Verification items for the finished model (mm, model axes). Face numbers are marked on the shaded views. A direction names the side the tool comes from. Round coordinates to 2 decimals unless told otherwise and drop trailing zeros. Loops run counter-clockwise (first coordinate to the right, second up) from the corner with the lowest first, then second, coordinate; pieces in that order, holes last. Notation, with made-up numbers: (57, -18.75) -> (74, -18.75) arc R4 cw to (74, -14.75) -> close; hole circle Ø4 at (34, -10). An arc over 180 degrees is marked (long way). Write item = value, one per line.
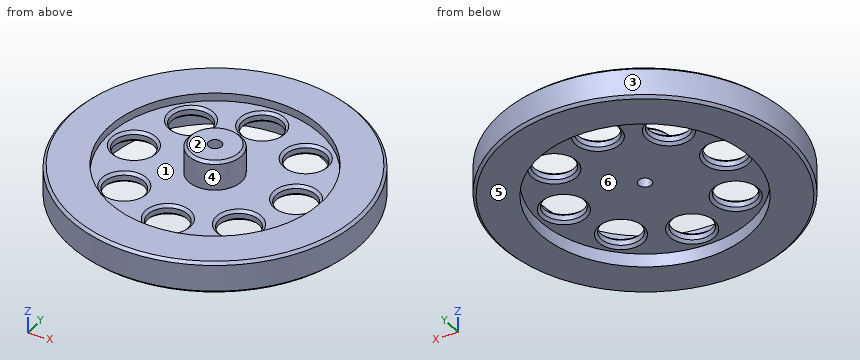
```python
from build123d import *

# Parameters (mm, degrees)
SKETCH1_R           = 55
BOSS_EXTRUDE1_DEPTH = 12
SKETCH2_R           = 40
CUT_EXTRUDE1_DEPTH  = 5
CUT_EXTRUDE2_START  = -3
SKETCH3_R           = 40
CUT_EXTRUDE2_DEPTH  = 3
SKETCH4_R           = 10
BOSS_EXTRUDE2_DEPTH = 11
SKETCH5_R           = 2.5
CUT_EXTRUDE3_DEPTH  = 81.311892021
SKETCH6_R           = 7.5
CUT_EXTRUDE4_DEPTH  = 79.555712714
CHAMFER1_SIZE       = 1


with BuildPart() as part:
    # Sketch1 → Boss-Extrude1 (new body)
    with BuildSketch(Plane.XY):
        Circle(SKETCH1_R)
    extrude(amount=BOSS_EXTRUDE1_DEPTH)

    # Sketch2 → Cut-Extrude1 (cut)
    with BuildSketch(Plane(origin=(0, 0, 0), x_dir=(-1, 0, 0), z_dir=(0, 0, -1))):
        Circle(SKETCH2_R)
    extrude(amount=-CUT_EXTRUDE1_DEPTH, mode=Mode.SUBTRACT)

    # Sketch3 → Cut-Extrude2 (cut)
    with BuildSketch(Plane.XY.offset(12).offset(CUT_EXTRUDE2_START)):
        with Locations(Location((0, 0, 0), (0, 0, 180))):
            Circle(SKETCH3_R)
    extrude(amount=CUT_EXTRUDE2_DEPTH, mode=Mode.SUBTRACT)

    # Sketch4 → Boss-Extrude2 (add)
    with BuildSketch(Plane.XY.offset(9)):
        Circle(SKETCH4_R)
    extrude(amount=BOSS_EXTRUDE2_DEPTH)

    # Sketch5 → Cut-Extrude3 (cut, through all)
    with BuildSketch(Plane.XY.offset(20)):
        Circle(SKETCH5_R)
    extrude(amount=-CUT_EXTRUDE3_DEPTH, mode=Mode.SUBTRACT)

    # Sketch6 → Cut-Extrude4 (cut, through all)
    with BuildSketch(Plane.XY.offset(9)):
        with Locations((0, 30)):
            Circle(SKETCH6_R)
        with Locations((21.213203436, 21.213203436)):
            Circle(SKETCH6_R)
        with Locations((30, 0)):
            Circle(SKETCH6_R)
        with Locations((21.213203436, -21.213203436)):
            Circle(SKETCH6_R)
        with Locations((0, -30)):
            Circle(SKETCH6_R)
        with Locations((-21.213203436, -21.213203436)):
            Circle(SKETCH6_R)
        with Locations((-30, 0)):
            Circle(SKETCH6_R)
        with Locations((-21.213203436, 21.213203436)):
            Circle(SKETCH6_R)
    extrude(amount=-CUT_EXTRUDE4_DEPTH, mode=Mode.SUBTRACT)

    # Chamfer1
    chamfer1_edges = [part.edges().sort_by_distance(p)[0] for p in [
        (-10, 0, 20),
        (-55, 0, 0),
        (-28.713203436, 21.213203436, 5),
        (-28.713203436, 21.213203436, 9),
        (-37.5, 0, 5),
        (-37.5, 0, 9),
        (-28.713203436, -21.213203436, 5),
        (-28.713203436, -21.213203436, 9),
        (-7.5, -30, 5),
        (-7.5, -30, 9),
        (13.713203436, -21.213203436, 5),
        (13.713203436, -21.213203436, 9),
        (22.5, 0, 5),
        (22.5, 0, 9),
        (13.713203436, 21.213203436, 5),
        (13.713203436, 21.213203436, 9),
        (-7.5, 30, 5),
        (-7.5, 30, 9),
        (-55, 0, 12),
    ]]
    chamfer(chamfer1_edges, length=CHAMFER1_SIZE)


solid = part.part
```
(1) Sectioned sample at B-B, the plane z = 16. Record the cut outline in (x, y).
Filled sheet:
outline = circle Ø20 at (0, 0); hole circle Ø5 at (0, 0)
(2) Draft check along X on the marked faces 1, 2, 3 and 4. Enter one of: released by +X, released by -X, zero draft, split by the parting line, or undercut.
Filled sheet:
face_1 = undercut
face_2 = zero draft
face_3 = split by the parting line
face_4 = undercut
(3) Set-up check for the marked faces 5 and 6: record each of +Z, -Z, +X, -X, +Y, -Y from which the full face is reachable in a straight line by a thin tool's end or side.
Filled sheet:
face_5 = -Z, +X, -X, +Y, -Y
face_6 = -Z
(4) Sectioned sample at A-A, the plane y = 0. Count the separate pieces of the cut face and the enclosed holes in it, and give its area (3 significant figures).
Filled sheet:
separate_pieces = 4
enclosed_holes = 0
area = 698 mm2
(5) Go/stop test with flat-tipped pins: pin 1 Ø2 at (x, z) = (-32.5, 6.5) entering from -Y; pin 2 Ø19.5 at (x, y) = (21.21, -21.21) entering from -Z; pin 3 Ø6 at (y, z) = (32, 2.5) entering from +X. Record where each tip stops, or that it passes through.
Filled sheet:
pin_1 = -45.09
pin_2 = 5
pin_3 = 46.73
(6) Material ranges on probe 1 along X at (y, z) = (20.5, 6); probe 2 along X at (y, z) = (-20, 7.25); probe 3 along Y at (x, z) = (0, 3.65), recorded low to high. Write a range as from..to.
Filled sheet:
probe_1 = -51.04..-28.68, -13.75..13.75, 28.68..51.04
probe_2 = -51.23..-28.61, -13.81..13.81, 28.61..51.23
probe_3 = -55..-40, 40..55
